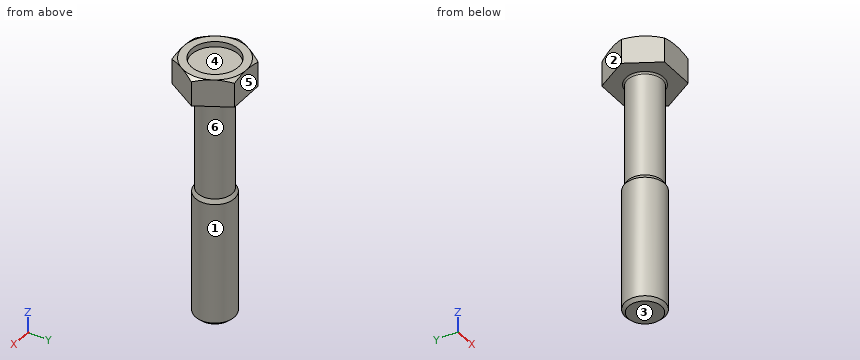
Autodesk Inventor part; units mm, degrees
ref_plane "MSC_PF1" through (0, 0, 0) normal (0, 1, 0) x (-1, 0, 0)
ref_plane "MSC_PT1" through (0, 0, -6.7108) normal (0, 0, -1) x (-1, 0, 0)
ref_plane "YZ Plane" through (0, 0, 0) normal (1, 0, 0) x (0, 1, 0)
sketch "Sketch2" plane through (0, 0, 0) normal (0, 1, 0) x (-1, 0, 0)
  line L0 (0, -6.7108) -> (0, -36.7108)
  line L1 (0, -36.7108) -> (2.1, -36.7108)
  line L2 (2.5, -36.3108) -> (2.5, -20.7108)
  line L3 (2.5, -20.7108) -> (2.2, -20.1912)
  line L4 (2.2, -20.1912) -> (2.2, -6.7108)
  line L5 (2.2, -6.7108) -> (0, -6.7108)
  line L6 (2.1, -36.7108) -> (2.5, -36.3108)
  line L7 (2.5, -36.7108) -> (2.5, -37.2765)
  line L8 (0, -43.3897) -> (0, -0.5977)
  dimension "Ds" = 4.4
  dimension "NND" = 5
  dimension "b" = 16
  dimension "d3" = 30
  dimension "d5" = 45
  dimension "PTC" = 0.8
  dimension "NLG" = 30
revolve "Revolution1" add sketch "Sketch2" angle 360 about axis through (0, 0, -6.7108) along (0, 0, -1)
sketch "Sketch3" plane through (0, 0, -6.7108) normal (0, 0, 1) x (1, 0, 0)
  circle A0 centre (0, 0) radius 2.2
  line L0 (0, 4) -> (2.3094, 4)
  line L1 (2.3094, 4) -> (4.6188, 0)
  line L2 (4.6188, 0) -> (0, 0)
  line L3 (0, 0) -> (0, 4)
  line L4 (0, 4) -> (-2.3094, 4)
  line L5 (-2.3094, 4) -> (-4.6188, 0)
  line L6 (0, -4) -> (2.3094, -4)
  line L7 (2.3094, -4) -> (4.6188, 0)
  line L8 (-2.3094, -4) -> (-4.6188, 0)
  line L9 (0, -4) -> (-2.3094, -4)
  dimension "d9" = 60
  dimension "ParS" = 8
  dimension "msp_d11" = 8
extrude "Extrusion1" add sketch "Sketch3" along normal blind 3.5
sketch "Sketch4" plane through (0, 0, 0) normal (0, 1, 0) x (-1, 0, 0)
  line L0 (-4, -3.2108) -> (-4.6188, -3.2108)
  line L1 (-4.6188, -3.2108) -> (-4.6188, -3.5681)
  line L2 (-4.6188, -3.5681) -> (-4, -3.2108)
  line L3 (0, -13.5602) -> (0, 34.3854)
  line L4 (0, 27.536) -> (0, 27.1787)
  line L5 (-4.6188, -6.7108) -> (-4.6188, -3.2108)
  line L6 (-2.3094, -3.2108) -> (-4.6188, -3.2108)
  dimension "d14" = 30
  dimension "msp_d15" = 8
revolve "Revolution2" cut sketch "Sketch4" angle 360 about axis through (0, 0, 27.536) along (0, 0, -1)
sketch "Sketch5" plane through (0, 0, -3.2108) normal (0, 0, 1) x (1, 0, 0)
  arc A0 (3.4641, 2) -> (0, 4) centre (0, 0) ccw
  circle A1 centre (0, 0) radius 3
  dimension "d27" = 6
extrude "Extrusion2" cut sketch "Sketch5" against normal blind 0.7
thread "Thread1"
ref_plane "MSC_PF1" through (0, 0, 0) normal (0, 1, 0) x (-1, 0, 0)
ref_plane "MSC_PT1" through (0, 0, -6.7108) normal (0, 0, -1) x (-1, 0, 0)
fillet "Fillet1" radius 0.2 1 edges at (2.2, 0, -6.7108)
equation "\"msp_d11\" = ParS"
equation "\"msp_d15\" = ParS"
equation "\"d27\" = 0.75 * ParS"
equation "\"d28\" = 0.2 * ParK"
equation "\"d30\" = r"
equation "\"msp_d17\" = b"
equation "\"r\" = 0.2"
equation "\"THREADDIA\" = NND"
properties part number "ISO 4015 - M5 x 30" material "Stainless Steel, 440C"
Work out the finished part from the listing and answer in its coordinate system (mm). Face numbers are marked on the shaded views. A direction names the side the tool comes from. Round coordinates to 2 decimals unless told otherwise and drop trailing zeros. Write each loop counter-clockwise with the first axis right and the second up, starting at its lowest first coordinate (ties: lowest second). Pieces come first, ordered by that corner, then holes. Notation, with made-up numbers: M 55,21 L 97,21 A18 ccw 97,32 Z; hole C 66,53 d10. An arc over 180 degrees is marked long. Use a Markdown table: item, result.
1) Flat-ended cylindrical pins translate along their axes: pin 1 (1 mm diameter, centred on x = 3, z = -16, fed in from +Y); pin 2 (3 mm diameter, centred on x = 2.5, y = 0.5, fed in from +Z); pin 3 (3 mm diameter, centred on x = 2.5, z = -29, fed in from -Y); pin 4 (2 mm diameter, centred on y = 1.5, z = -7.5, fed in from +X). Find the tip coordinate at first contact, or state that the pin passes through.
Taken from the geometry:
| item | result |
|---|---|
| pin 1 | passes through |
| pin 2 | stops at z = -3.21 |
| pin 3 | stops at y = -2.29 |
| pin 4 | stops at x = 4.11 |
2) Which of the six approach directions +Z, -Z, +X, -X, +Y, -Y give full straight-line access (tool end or side, diameter ignored) to the marked faces 1 and 2?
Taken from the geometry:
| item | result |
|---|---|
| face 1 | -Z |
| face 2 | +Z, -Z, -X, +Y |
3) Determine the mould class of the marked faces 3, 4, 5 and 6 for opening direction Z: pulls with the +Z half, pulls with the -Z half, needs draft (parallel to the pull), parting line crosses it, or undercut.
Taken from the geometry:
| item | result |
|---|---|
| face 3 | pulls with the -Z half |
| face 4 | pulls with the +Z half |
| face 5 | needs draft |
| face 6 | undercut |
4) Consider line 1 (Z direction, x = -1.25, y = 1); line 2 (Y direction, x = 0, z = -3.55); line 3 (Z direction, x = 1.25, y = 3.5). Determine where each line is inside the solid, lowest interval first. Write a range as [from, to].
Taken from the geometry:
| item | result |
|---|---|
| line 1 | z = [-36.71, -3.91] |
| line 2 | y = [-4, -3], [3, 4] |
| line 3 | z = [-6.71, -3.21] |
5) The part is cut by section A-A on z = -24. Give the vertices of the cut face in (x, y).
Taken from the geometry:
| item | result |
|---|---|
| outline | C 0,0 d5 |
6) The part is cut by section B-B on z = -9. Give the vertices of the cut face in (x, y).
Taken from the geometry:
| item | result |
|---|---|
| outline | C 0,0 d4.4 |
